Read the model definition and answer for the solid it produces. Units are mm, in the model's axes. A direction names the side the tool comes from. Give positions to 0.01 mm unless a question says otherwise; leave off trailing zeros. Order: outer loops, then holes, each group sorted by start corner. A loop starts at its lowest first (then second) coordinate and runs counter-clockwise, first axis right, second up.
```python
from build123d import *

# Parameters (mm, degrees)
F0_W           = 36
F0_H           = 18
F1_DEPTH       = 15
F3_DEPTH       = 18
F4_DEPTH       = 15
F5_SIZE        = 5
F6_D           = 3.5
F6_CBORE_D     = 10
F6_CBORE_DEPTH = 20


# Not quite as in the source:
# - a feature names something its author has since deleted; it is built from what else it names


with BuildPart() as f1:
    # F0 (on Top) → F1 (new body)
    with BuildSketch(Plane.XY):
        with Locations((0, -9)):
            Rectangle(F0_W, F0_H)
    extrude(amount=F1_DEPTH)

    # F2 (on Front) → F3 (join)
    with BuildSketch(Plane.XZ):
        Polygon((-17.9443880916, 0), (-18, 15), (-41.1238394028, 30.7888584537), (-41.1238394028, 25.5634840578), (-28.7360682942, 17.105167029), (-28.7360682942, 13.1013058126), (-41.1238394028, 21.5596228414), (-41.1238394028, 15.7888584537), align=None)
        Polygon((28.7360682942, 17.105167029), (41.1238394028, 25.5634840578), (41.1238394028, 30.7888584537), (18, 15), (17.9443880916, 0), (41.1238394028, 15.7888584537), (41.1238394028, 21.5596228414), (28.7360682942, 13.1013058126), align=None)
    extrude(amount=F3_DEPTH)

    # F4 (add): a face of the model
    f4_faces = [f1.faces().sort_by_distance(p)[0] for p in [
        (0, -9, 15),
    ]]
    extrude(f4_faces, amount=F4_DEPTH)

    # F5
    f5_edges = [f1.edges().sort_by_distance(p)[0] for p in [
        (41.123839, -9, 30.788858),
        (-41.123839, -9, 30.788858),
    ]]
    chamfer(f5_edges, length=F5_SIZE)

    # F6 (through all)
    with Locations(Plane(origin=(0, 0, 0), x_dir=(1, 0, 0), z_dir=(0, 0, -1))):
        with Locations((-10, 10), (10, 10)):
            CounterBoreHole(F6_D / 2, F6_CBORE_D / 2, F6_CBORE_DEPTH)


solid = f1.part
```
1) Consider L1, parallel to Y at x = 10, z = 11.25; L2, parallel to Y at x = -10, z = 25.75; L3, parallel to X at y = -9, z = 26.25. Determine where each line is inside the solid, lowest interval first.
Final values:
L1: y = -18 to -15, -5 to 0
L2: y = -18 to -11.75, -8.25 to 0
L3: x = -40.25 to -34.48, -18 to -11.44, -8.56 to 8.56, 11.44 to 18, 34.48 to 40.25
2) The part is cut by section A-A on x = 10. Determine the outline of the cut face in (y, z).
Final values:
outline: (-18, 0) - (-15, 0) - (-15, 20) - (-11.75, 20) - (-11.75, 30) - (-18, 30) - close; (-8.25, 20) - (-5, 20) - (-5, 0) - (0, 0) - (0, 30) - (-8.25, 30) - close
3) The part is cut by section D-D on z = 19.25. Determine the outline of the cut face in (x, y).
Final values:
outline: (-41.12, -18) - (-37.74, -18) - (-37.74, 0) - (-41.12, 0) - close; (-31.88, -18) - (-24.22, -18) - (-24.22, 0) - (-31.88, 0) - close; (-18, -18) - (18, -18) - (18, 0) - (-18, 0) - close; (24.22, -18) - (31.88, -18) - (31.88, 0) - (24.22, 0) - close; (37.74, -18) - (41.12, -18) - (41.12, 0) - (37.74, 0) - close; hole circle Ø10 at (-10, -10); hole circle Ø10 at (10, -10)
4) For a pull along X with two mould halves and no side action, classify faces 1 (the face through (34.843, -8.874, 21.275)), 2 (the face through (-29.72, -8.87, 8.02)), 3 (the face through (-1, 0, 15)) as released by +X, released by -X, zero draft, split by the parting line, or undercut.
Final values:
face 1: undercut
face 2: released by -X
face 3: zero draft
5) The part is cut by section B-B on z = 24. Determine the outline of the cut face in (x, y), and give its area (3 significant figures).
Final values:
outline: (-38.83, -18) - (-31.18, -18) - (-31.18, 0) - (-38.83, 0) - close; (-18, -18) - (18, -18) - (18, 0) - (-18, 0) - close; (31.18, -18) - (38.83, -18) - (38.83, 0) - (31.18, 0) - close; hole circle Ø3.5 at (-10, -10); hole circle Ø3.5 at (10, -10)
area: 904 mm2
6) A tool of negligible diameter and unlimited length cuts with its end or side. For faces 4 (the face through (-27.36, -8.87, 21.39)), 5 (the face through (-34.84, -8.87, 17.27)), 6 (the face through (29.4, -8.874, 7.803)), 7 (the face through (14.77, -11.5, 9.86)), from which of +Z, -Z, +X, -X, +Y, -Y can it reach the whole face along a straight path? Write none if from no direction.
Final values:
face 4: +Z, +Y, -Y
face 5: +Y, -Y
face 6: -Z, +X, +Y, -Y
face 7: -Z
7) Given pin 1 (2 mm diameter, centred on y = -10, z = 24.5, fed in from -X); pin 2 (3 mm diameter, centred on x = 10, y = -10, fed in from -Z); pin 3 (1.5 mm diameter, centred on x = 19.5, y = -5, fed in from +Z); pin 4 (4 mm diameter, centred on x = -10, y = -10, fed in from -Z), each flat-ended and moving along its own axis, determine where each tip first touches the part or whether it passes through.
Final values:
pin 1: stops at x = -41.03
pin 2: passes through
pin 3: stops at z = 16.54
pin 4: stops at z = 20
